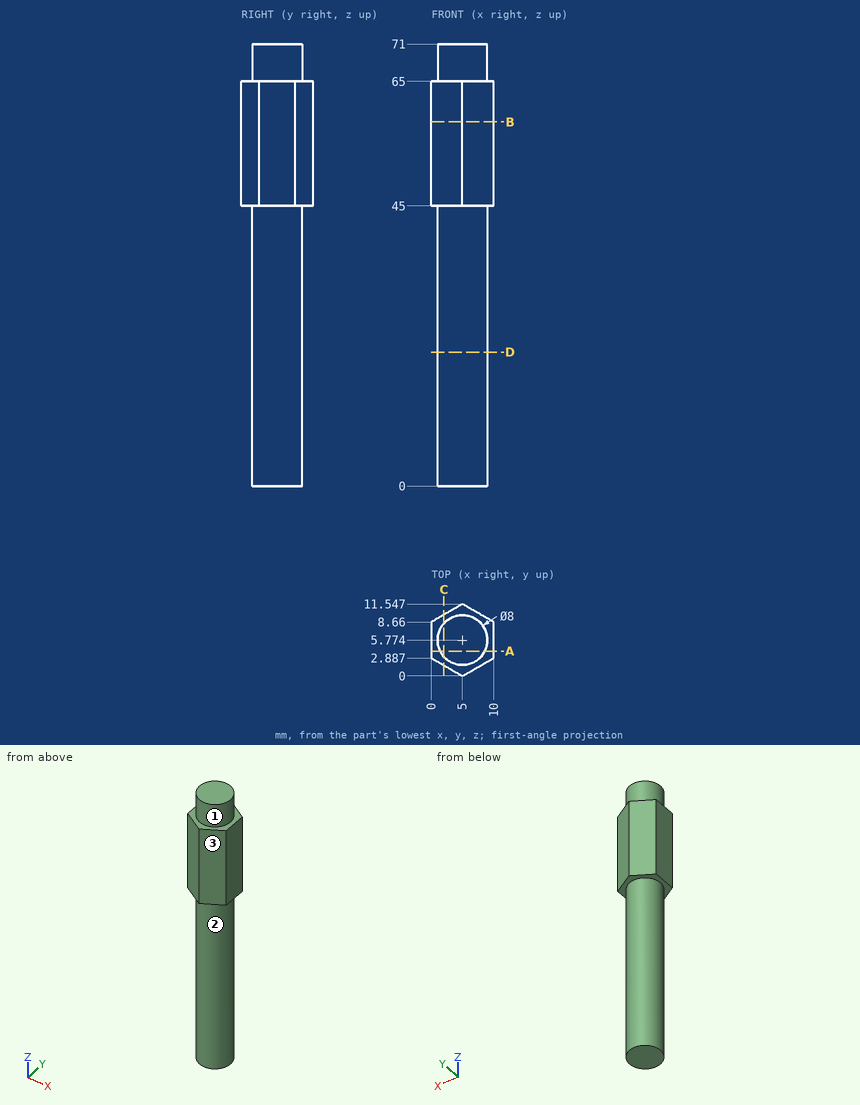
Answer from the drawing. Dimensions are ordinates in mm from the lowest x, y and z of the part. A direction names the side the tool comes from. Coordinates: 2 decimals unless noted, no trailing zeros. Write each loop counter-clockwise with the first axis right and the second up, starting at its lowest first coordinate (ties: lowest second). Pieces come first, ordered by that corner, then holes. Notation, with made-up numbers: (67, 3) - (110, 3) arc R22 ccw to (110, 18) - close; hole circle Ø8 at (54, -12.75). An arc over 180 degrees is marked (long way). Return JSON: item names as keys, results as strings.
1. The part is cut by section B-B on z = 58.5. Determine the outline of the cut face in (x, y).
Final values:
{"outline": "(0, 2.89) - (5, 0) - (10, 2.89) - (10, 8.66) - (5, 11.55) - (0, 8.66) - close"}
2. The part is cut by section D-D on z = 21.5. Determine the outline of the cut face in (x, y).
Final values:
{"outline": "circle Ø8 at (5, 5.77)"}
3. Consider line 1 along Z through (x, y) = (8, 9.5); line 2 along Y through (x, z) = (4.75, 29) (1 decimal); line 3 along Y through (x, z) = (3.75, 25) (1 decimal). Determine where each line is inside the solid, lowest interval first.
Final values:
{"line 1": "45 to 65", "line 2": "1.8 to 9.8", "line 3": "2 to 9.6"}
4. Which of the six approach directions +Z, -Z, +X, -X, +Y, -Y give full straight-line access (tool end or side, diameter ignored) to the marked faces 1, 2 and 3?
Final values:
{"face 1": "+Z", "face 2": "-Z", "face 3": "+Z, -Z, +X, -Y"}
5. The part is cut by section A-A on y = 4. Determine the outline of the cut face in (x, z) (1 decimal).
Final values:
{"outline": "(0, 45) - (1.4, 45) - (1.4, 0) - (8.6, 0) - (8.6, 45) - (10, 45) - (10, 65) - (8.6, 65) - (8.6, 71) - (1.4, 71) - (1.4, 65) - (0, 65) - close"}
6. The part is cut by section C-C on x = 2. Determine the outline of the cut face in (y, z) (1 decimal).
Final values:
{"outline": "(1.7, 45) - (3.1, 45) - (3.1, 0) - (8.4, 0) - (8.4, 45) - (9.8, 45) - (9.8, 65) - (8.4, 65) - (8.4, 71) - (3.1, 71) - (3.1, 65) - (1.7, 65) - close"}
7. Each of these flat-tipped pins is pushed along its axis until it touches: pin 1 Ø3 at (x, z) = (7, 37) entering from +Y; pin 2 Ø3 at (x, z) = (1.5, 20.5) entering from -Y. Where does it stop, or does it pass through?
Final values:
{"pin 1": "y = 9.74", "pin 2": "y = 2.31"}
